```python
from build123d import *

# Parameters (mm, degrees)
SKETCH_1_R      = 1.75
EXTRUDE_1_DEPTH = 6
CHAMFER_1_SIZE  = 0.5
SKETCH_2_R      = 5.5
EXTRUDE_2_DEPTH = 10


with BuildPart() as part:
    # 草图1 → 凸台-拉伸1 (new body)
    with BuildSketch(Plane.XY):
        Polygon((3.464101615, 6), (-3.464101615, 6), (-6.92820323, 0), (-3.464101615, -6), (3.464101615, -6), (6.92820323, 0), align=None)
        Circle(SKETCH_1_R, mode=Mode.SUBTRACT)
    extrude(amount=EXTRUDE_1_DEPTH)

    # 倒角1
    chamfer_1_edges = [part.edges().sort_by_distance(p)[0] for p in [
        (-5.196152423, 3, 6),
        (-5.196152423, -3, 6),
        (0, -6, 6),
        (5.196152423, -3, 6),
        (5.196152423, 3, 6),
        (5.196152423, -3, 0),
        (0, -6, 0),
        (-5.196152423, -3, 0),
        (-5.196152423, 3, 0),
        (0, 6, 0),
        (5.196152423, 3, 0),
        (0, 6, 6),
    ]]
    chamfer(chamfer_1_edges, length=CHAMFER_1_SIZE)

    # 草图2 → 凸台-拉伸2 (add)
    with BuildSketch(Plane.XY.offset(6)):
        with Locations(Location((0, 0, 0), (0, 0, 150))):
            Circle(SKETCH_2_R)
        with BuildLine():
            Line((-1.5, 2), (1.5, 2))
            ThreePointArc((1.5, 2), (0, -2.5), (-1.5, 2))
        make_face(mode=Mode.SUBTRACT)
    extrude(amount=EXTRUDE_2_DEPTH)


solid = part.part
```
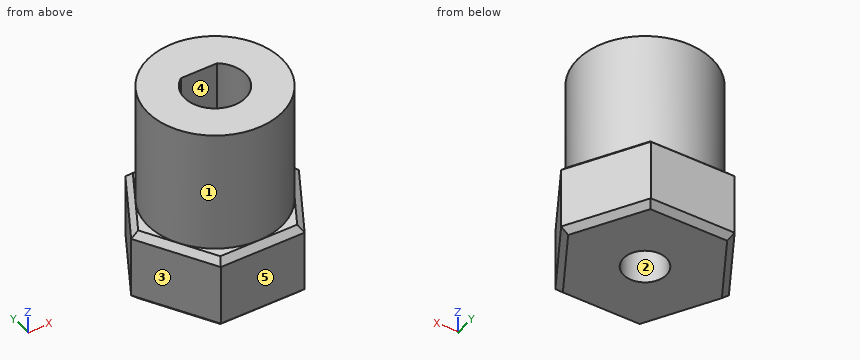
The model under review builds one solid part; all positions refer to its coordinate system, in mm. Face numbers are marked on the shaded views. A direction names the side the tool comes from. Round coordinates to 2 decimals unless told otherwise and drop trailing zeros. Write each loop counter-clockwise with the first axis right and the second up, starting at its lowest first coordinate (ties: lowest second). Pieces come first, ordered by that corner, then holes. Notation, with made-up numbers: M 70,18 L 90,18 A12 ccw 90,27 Z; hole C 5,25.25 d1. An arc over 180 degrees is marked long. Use CSV: the item, a comma, the result in double quotes. Start each with the question number.
(1) The part is to be moulded in two halves that separate along Y. For the marked faces 1, 2 and 3, say which applies: +Y half, -Y half, draft (parallel to the pull), parting line (faces both ways), or undercut.
(2) We need section A-A, the plane z = 3.75. State the section outline as (x, y) points, then the cut area to 3 significant figures.
(3) We need section B-B, the plane x = -0.75. State the section outline as (y, z) points, then the cut area to 3 significant figures.
(4) Clearance check with flat-ended pins moving along their axes: P1, Ø3.5, axis at x = 0.5, z = 9.5, coming from the -Y side; P2, Ø3, axis at x = -4, z = 9, coming from the -Y side; P3, Ø5, axis at x = 3.5, z = 9, coming from the +Y side; P4, Ø6, axis at x = 0, y = 0, coming from the -Z side. State where each tip first meets the part, or that it passes through.
(5) For line 1 along X through (y, z) = (0, 13); line 2 along Y through (x, z) = (0, 1.55); line 3 along Y through (x, z) = (0, 12.5), list the stretches that pass through material, from the lowest coordinate up.
(6) Tool access review of the marked faces 4 and 5: name each direction out of +Z, -Z, +X, -X, +Y, -Y from which nothing blocks a thin tool from reaching the whole face with its end or side.
(7) We need section D-D, the plane x = 5. State the section outline as (y, z) points, then the cut area to 3 significant figures.
Findings:
1,face 1,"parting line"
1,face 2,"undercut"
1,face 3,"-Y half"
2,outline,"M -6.93,0 L -3.46,-6 L 3.46,-6 L 6.93,0 L 3.46,6 L -3.46,6 Z; hole C 0,0 d3.5"
2,area,"115 mm^2"
3,outline,"M -6,0.5 L -5.5,0 L -1.58,0 L -1.58,6 L -2.38,6 L -2.38,16 L -5.45,16 L -5.45,6 L -5.5,6 L -6,5.5 Z; M 1.58,0 L 5.5,0 L 6,0.5 L 6,5.5 L 5.5,6 L 5.45,6 L 5.45,16 L 2,16 L 2,6 L 1.58,6 Z"
3,area,"118 mm^2"
4,P1,"y = -5.5"
4,P2,"y = -4.9"
4,P3,"y = 5.41"
4,P4,"z = 0"
5,line 1,"-5.5 to -2.5, 2.5 to 5.5"
5,line 2,"-6 to -1.75, 1.75 to 6"
5,line 3,"-5.5 to -2.5, 2 to 5.5"
6,face 4,"+Z"
6,face 5,"+Z, -Z, +X, -X, -Y"
7,outline,"M -3.34,0.5 L -2.34,0 L 2.34,0 L 3.34,0.5 L 3.34,5.5 L 2.34,6 L 2.29,6 L 2.29,16 L -2.29,16 L -2.29,6 L -2.34,6 L -3.34,5.5 Z"
7,area,"84.9 mm^2"
